Print and shaded views of the part. All mm, measured from the part's lowest x, y and z. A direction names the side the tool comes from. Coordinates: 2 decimals unless noted, no trailing zeros. Loops run counter-clockwise (first coordinate to the right, second up) from the corner with the lowest first, then second, coordinate; pieces in that order, holes last. Notation, with made-up numbers: M -6,81 L 11,81 A14 cw 11,86 Z; hole C 10,-4.5 d8. An arc over 180 degrees is marked long. Use a Markdown table: item, result. Add a question column.
1) Tool access for the marked faces 1, 2, 3, 4 and 5: list every direction of +Z, -Z, +X, -X, +Y, -Y with a clear straight run to the whole face (end or side of a thin tool).
2) Band-saw the part on D-D (z = 28). List the corners of the cut face in (x, y), plus the area to 3 significant figures.
3) Band-saw the part on A-A (x = 65). List the corners of the cut face in (y, z).
4) Pin check, flat tips, straight feed: pin 1 Ø8 at (x, y) = (61, 45) entering from +Z; pin 2 Ø1.5 at (x, z) = (52, 1.5) entering from +Y; pin 3 Ø12.5 at (x, z) = (29.5, 20) entering from +Y. Stop position of each tip, or through.
5) Band-saw the part on B-B (y = 24). List the corners of the cut face in (x, z).
6) Band-saw the part on C-C (y = 30.5). List the corners of the cut face in (x, z) (1 decimal), plus the area to 3 significant figures.
7) Pull direction Y, two halves, no side cores. Call the marked faces 6, 7 and 8: released by +Y, released by -Y, zero draft, split by the parting line, or undercut.
8) Wall check: probe 1 along Z at (x, y) = (36.5, 33.5); probe 2 along X at (y, z) = (16, 37.5) (1 decimal); probe 3 along X at (y, z) = (35, 8.75). Give the ranges that are in metal, low to high. Write a range as from..to.
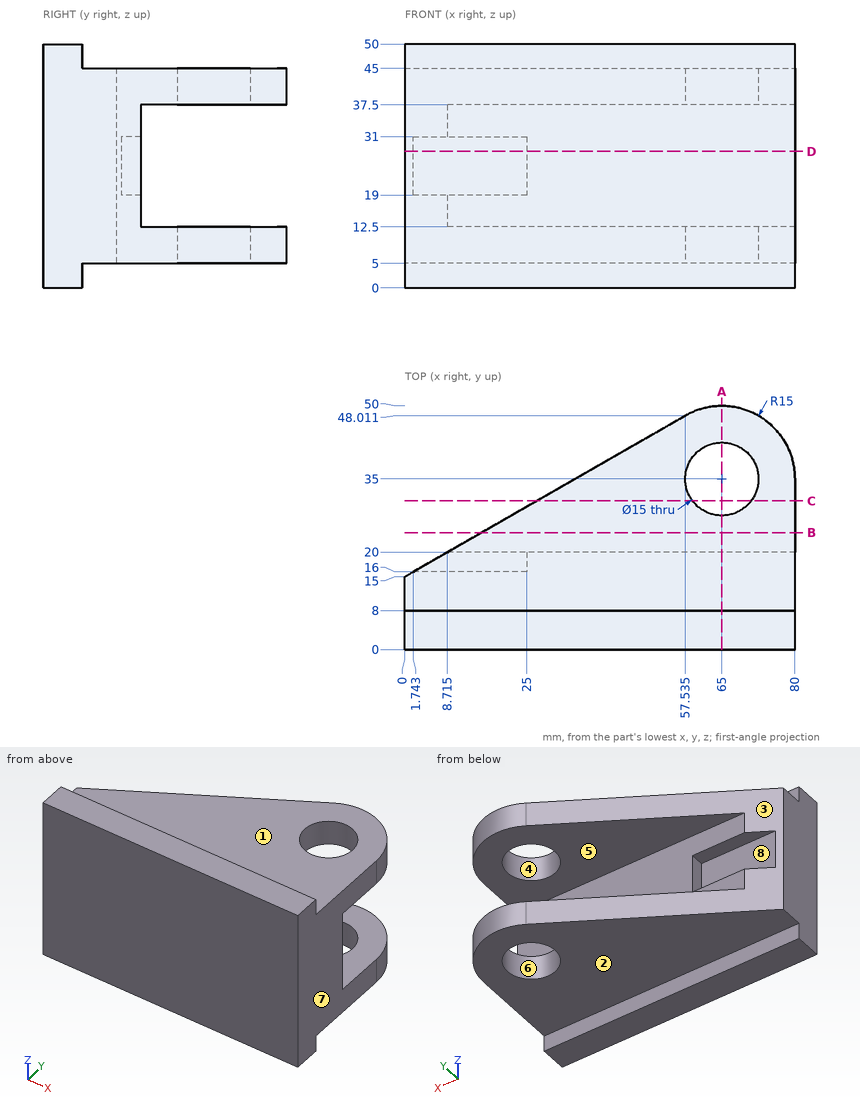
Entries:
| question | item | result |
|---|---|---|
| 1 | face 1 | +Z, +X, -X, +Y |
| 1 | face 2 | -Z, +X, -X, +Y |
| 1 | face 3 | +Z, -Z, -X, +Y |
| 1 | face 4 | +Z, -Z |
| 1 | face 5 | +X, -X, +Y |
| 2 | outline | M 0,0 L 80,0 L 80,20 L 25,20 L 25,16 L 1.74,16 L 0,15 Z |
| 2 | area | 1,500 mm2 |
| 3 | outline | M 0,0 L 8,0 L 8,5 L 27.5,5 L 27.5,12.5 L 20,12.5 L 20,37.5 L 27.5,37.5 L 27.5,45 L 8,45 L 8,50 L 0,50 Z; M 42.5,5 L 50,5 L 50,12.5 L 42.5,12.5 Z; M 42.5,37.5 L 50,37.5 L 50,45 L 42.5,45 Z |
| 4 | pin 1 | z = 45 |
| 4 | pin 2 | y = 8 |
| 4 | pin 3 | y = 20 |
| 5 | outline | M 15.69,5 L 80,5 L 80,12.5 L 15.69,12.5 Z; M 15.69,37.5 L 80,37.5 L 80,45 L 15.69,45 Z |
| 6 | outline | M 27,5 L 59,5 L 59,12.5 L 27,12.5 Z; M 27,37.5 L 59,37.5 L 59,45 L 27,45 Z; M 71,5 L 80,5 L 80,12.5 L 71,12.5 Z; M 71,37.5 L 80,37.5 L 80,45 L 71,45 Z |
| 6 | area | 615 mm2 |
| 7 | face 6 | undercut |
| 7 | face 7 | zero draft |
| 7 | face 8 | released by +Y |
| 8 | probe 1 | 5..12.5, 37.5..45 |
| 8 | probe 2 | 1.7..80 |
| 8 | probe 3 | 34.86..57.5, 72.5..80 |
